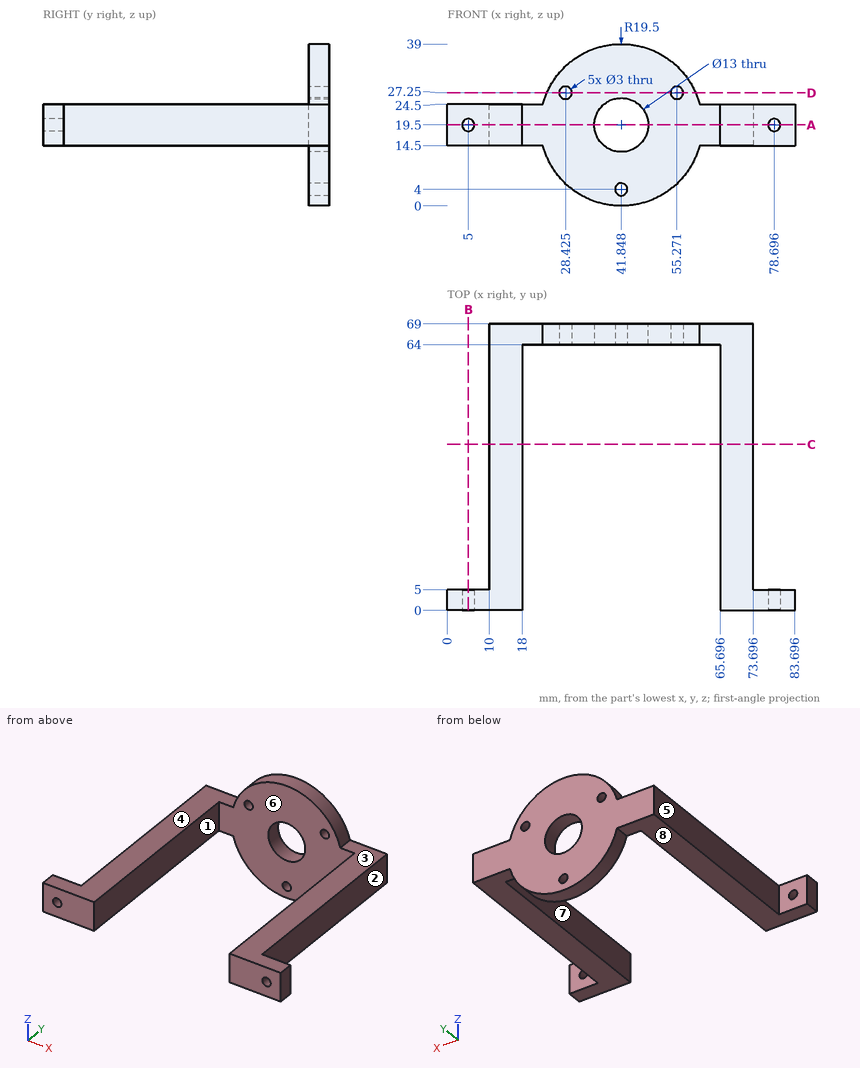
Can you work these out from the drawing? Everything is in mm from the part's minimum corner. A direction names the side the tool comes from. Coordinates: 2 decimals unless noted, no trailing zeros. Loops run counter-clockwise (first coordinate to the right, second up) from the corner with the lowest first, then second, coordinate; pieces in that order, holes last.
1. Imagine slicing it at C-C, the plane y = 40. Please give me the cut outline in (x, z), and give its area (3 significant figures).
2. I need wall thicknesses on L1, parallel to X at y = 15, z = 23.5; L2, parallel to X at y = 65.75, z = 27.25 (1 decimal); L3, parallel to Z at x = 17, y = 20. Which ranges of each line are inside material? Lowest first, please.
3. If we mould it in two halves opening along X, with no side actions, what happens to the marked faces 5, 6, 7 and 8? For each: pulls with the +X half, pulls with the -X half, needs draft (parallel to the pull), parting line crosses it, or undercut.
4. Imagine slicing it at A-A, the plane z = 19.5. Please give me the cut outline in (x, y), and give its area (3 significant figures).
5. For the marked faces 1, 2, 3 and 4, which set-ups out of +Z, -Z, +X, -X, +Y, -Y let a thin tool reach every point of the face, with its end or its side?
6. Imagine slicing it at D-D, the plane z = 27.25. Please give me the cut outline in (x, y) (1 decimal).
7. Imagine slicing it at B-B, the plane x = 5. Please give me the cut outline in (y, z), and give its area (3 significant figures).
8. For P1, Ø10, axis at y = 24.5, z = 16, coming from the +X side; P2, Ø8, axis at x = 79, z = 19, coming from the +Y side; P3, Ø3.5, axis at x = 41.85, z = 4, coming from the -Y side; P4, Ø1.8, axis at x = 28.42, z = 27.25, coming from the +Y side, each with a flat end and sliding along its axis, tell me the tip position at first contact or that it passes through.
Taken from the geometry:
1. outline: (10, 14.5) - (18, 14.5) - (18, 24.5) - (10, 24.5) - close; (65.7, 14.5) - (73.7, 14.5) - (73.7, 24.5) - (65.7, 24.5) - close
1. area: 160 mm2
2. L1: x = 10 to 18, 65.7 to 73.7
2. L2: x = 24 to 26.9, 29.9 to 53.8, 56.8 to 59.7
2. L3: z = 14.5 to 24.5
3. face 5: pulls with the -X half
3. face 6: undercut
3. face 7: undercut
3. face 8: needs draft
4. outline: (0, 0) - (3.5, 0) - (3.5, 5) - (0, 5) - close; (6.5, 0) - (18, 0) - (18, 64) - (35.35, 64) - (35.35, 69) - (10, 69) - (10, 5) - (6.5, 5) - close; (48.35, 64) - (65.7, 64) - (65.7, 0) - (77.2, 0) - (77.2, 5) - (73.7, 5) - (73.7, 69) - (48.35, 69) - close; (80.2, 0) - (83.7, 0) - (83.7, 5) - (80.2, 5) - close
4. area: 1,350 mm2
5. face 1: +Z, -Z, -Y
5. face 2: +Z, -Z, +X, +Y
5. face 3: +Z, +X, +Y, -Y
5. face 4: +Z, -X, +Y, -Y
6. outline: (24, 64) - (26.9, 64) - (26.9, 69) - (24, 69) - close; (29.9, 64) - (53.8, 64) - (53.8, 69) - (29.9, 69) - close; (56.8, 64) - (59.7, 64) - (59.7, 69) - (56.8, 69) - close
7. outline: (0, 14.5) - (5, 14.5) - (5, 18) - (0, 18) - close; (0, 21) - (5, 21) - (5, 24.5) - (0, 24.5) - close
7. area: 35.0 mm2
8. P1: stops at x = 73.7
8. P2: stops at y = 5
8. P3: stops at y = 64
8. P4: passes through
